Can you work these out from the drawing? Everything is in mm from the part's minimum corner. A direction names the side the tool comes from. Coordinates: 2 decimals unless noted, no trailing zeros. Loops run counter-clockwise (first coordinate to the right, second up) from the corner with the lowest first, then second, coordinate; pieces in that order, holes last.
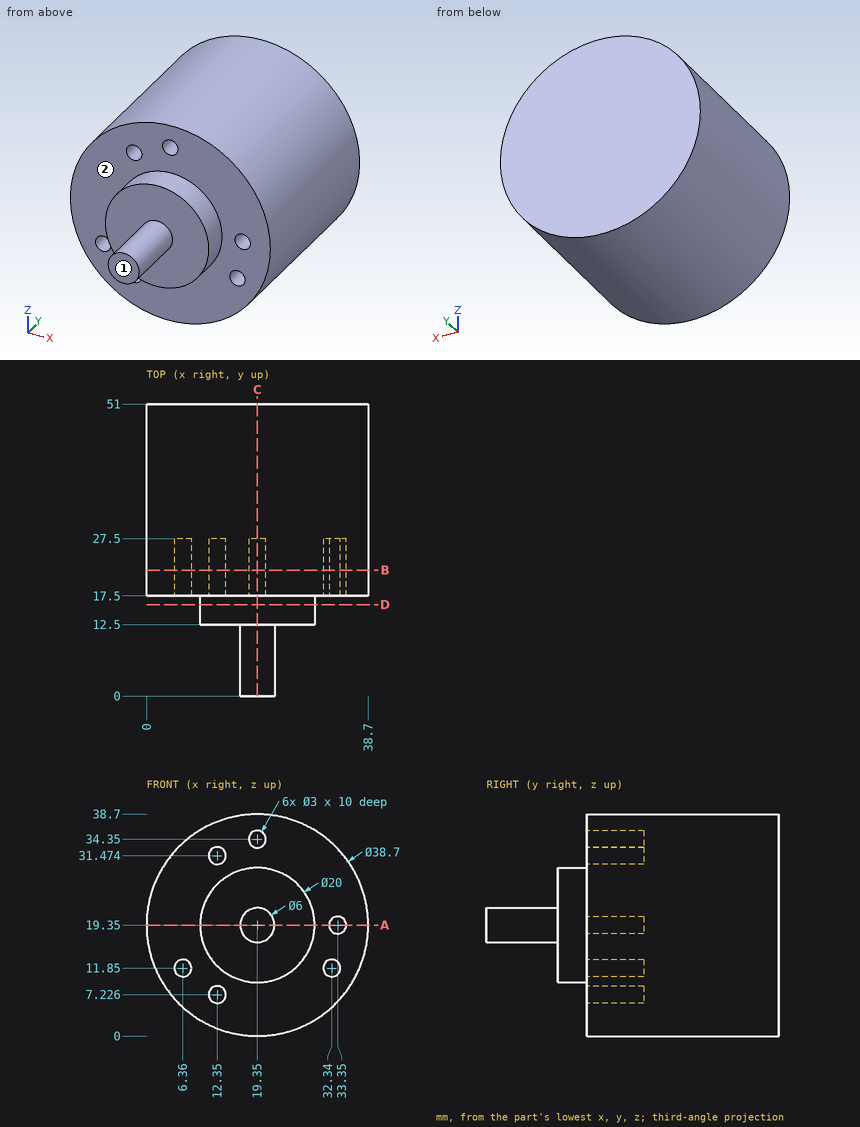
(1) Imagine slicing it at A-A, the plane z = 19.35. Write out the boundary of the cut face in (x, y).
Answers:
outline: (0, 17.5) - (9.35, 17.5) - (9.35, 12.5) - (16.35, 12.5) - (16.35, 0) - (22.35, 0) - (22.35, 12.5) - (29.35, 12.5) - (29.35, 17.5) - (31.85, 17.5) - (31.85, 27.5) - (34.85, 27.5) - (34.85, 17.5) - (38.7, 17.5) - (38.7, 51) - (0, 51) - close
(2) Which directions (+Z, -Z, +X, -X, +Y, -Y) give clear straight access to the entire face, cutting with the end or side of a thin tool? Please do the marked faces 1 and 2.
Answers:
face 1: +Z, -Z, +X, -X, -Y
face 2: -Y
(3) For pin 1 (2 mm diameter, centred on x = 15.5, z = 23.5, fed in from -Y); pin 2 (1.5 mm diameter, centred on x = 11.5, z = 32, fed in from -Y); pin 3 (0.9 mm diameter, centred on x = 33.5, z = 19, fed in from -Y), each with a flat end and sliding along its axis, tell me the tip position at first contact or that it passes through.
Answers:
pin 1: stops at y = 12.5
pin 2: stops at y = 17.5
pin 3: stops at y = 27.5
(4) I need wall thicknesses on probe 1 along Z at (x, y) = (32, 20) (1 decimal); probe 2 along Y at (x, z) = (7, 12); probe 3 along Y at (x, z) = (8, 13.5). Which ranges of each line are inside material? Lowest first, please.
Answers:
probe 1: z = 4.7 to 10.4, 13.3 to 18.7, 20 to 34
probe 2: y = 27.5 to 51
probe 3: y = 17.5 to 51
(5) Imagine slicing it at C-C, the plane x = 19.35. Write out the boundary of the cut face in (y, z).
Answers:
outline: (0, 16.35) - (12.5, 16.35) - (12.5, 9.35) - (17.5, 9.35) - (17.5, 0) - (51, 0) - (51, 38.7) - (17.5, 38.7) - (17.5, 35.85) - (27.5, 35.85) - (27.5, 32.85) - (17.5, 32.85) - (17.5, 29.35) - (12.5, 29.35) - (12.5, 22.35) - (0, 22.35) - close
(6) Imagine slicing it at B-B, the plane y = 22. State how many separate pieces and enclosed holes the cut face has, and give its area (3 significant figures).
Answers:
separate pieces: 1
enclosed holes: 6
area: 1,130 mm2
(7) Imagine slicing it at D-D, the plane y = 16. Write out the boundary of the cut face in (x, z).
Answers:
outline: circle Ø20 at (19.35, 19.35)
